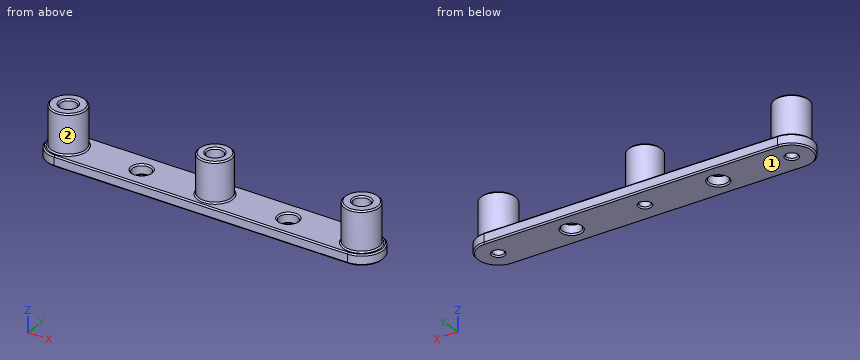
```python
from build123d import *

# Parameters (mm, degrees)
F0_R     = 3.5
F1_DEPTH = 4
F2_R     = 6.5
F2_R_2   = 6.15
F3_DEPTH = 15
F4_R     = 2
F5_DEPTH = 25
F6_R     = 3.05
F7_DEPTH = 6
F8_SIZE  = 0.5


with BuildPart() as f1:
    # F0 (on Top) → F1 (new body)
    with BuildSketch(Plane.XY):
        with BuildLine():
            Line((-56, -8), (56, -8))
            ThreePointArc((56, -8), (64, 0), (56, 8))
            Line((56, 8), (-56, 8))
            ThreePointArc((-56, 8), (-64, 0), (-56, -8))
        make_face()
        with Locations((-28, 0)):
            Circle(F0_R, mode=Mode.SUBTRACT)
        with Locations((28, 0)):
            Circle(F0_R, mode=Mode.SUBTRACT)
    extrude(amount=F1_DEPTH)

    # F2 (on face) → F3 (join)
    with BuildSketch(Plane.XY.offset(4)):
        with Locations((-56, 0)):
            Circle(F2_R)
        with Locations((56, 0)):
            Circle(F2_R)
        Circle(F2_R_2)
    extrude(amount=F3_DEPTH)

    # F4 (on face) → F5 (cut)
    with BuildSketch(Plane.XY.offset(19)):
        with Locations((56, 0)):
            Circle(F4_R)
        Circle(F4_R)
        with Locations((-56, 0)):
            Circle(F4_R)
    extrude(amount=-F5_DEPTH, mode=Mode.SUBTRACT)

    # F6 (on face) → F7 (cut)
    with BuildSketch(Plane.XY.offset(19)):
        with Locations((-56, 0)):
            Circle(F6_R)
        Circle(F6_R)
        with Locations((56, 0)):
            Circle(F6_R)
    extrude(amount=-F7_DEPTH, mode=Mode.SUBTRACT)

    # F8
    f8_edges = [f1.edges().sort_by_distance(p)[0] for p in [
        (-62.5, 0, 19),
        (-59.05, 0, 19),
        (-6.15, 0, 19),
        (-3.05, 0, 19),
        (49.5, 0, 19),
        (52.95, 0, 19),
        (-64, 0, 4),
        (0, 8, 4),
        (0, -8, 4),
        (64, 0, 4),
        (-62.5, 0, 4),
        (-31.5, 0, 4),
        (-6.15, 0, 4),
        (24.5, 0, 4),
        (49.5, 0, 4),
        (-64, 0, 0),
        (0, 8, 0),
        (0, -8, 0),
        (64, 0, 0),
        (-58, 0, 0),
        (-31.5, 0, 0),
        (-2, 0, 0),
        (24.5, 0, 0),
        (54, 0, 0),
        (-58, 0, 13),
        (-2, 0, 13),
        (54, 0, 13),
    ]]
    chamfer(f8_edges, length=F8_SIZE)


solid = f1.part
```
Source: CAD feature listing. Evaluate the final solid. Frame: model axes, mm. Face numbers are marked on the shaded views. Coordinates: 2 decimals unless noted, no trailing zeros. Loops run counter-clockwise (first coordinate to the right, second up) from the corner with the lowest first, then second, coordinate; pieces in that order, holes last. Notation, with made-up numbers: (32.25, -8) -> (87.25, -8) arc R15 cw to (87.25, 2) -> close; hole circle Ø11 at (62, 9). An arc over 180 degrees is marked (long way). One line per item, written item: value. Start each with the question number.
Q1. Section query C-C, the plane y = 0. Give the number of separate pieces and of enclosed holes in the cut face, and give its area (3 significant figures).
Q2. Line query: line 1 along Y through (x, z) = (-28, 2.25); line 2 along Y through (x, z) = (-56, 15); line 3 along X through (y, z) = (4, 14.5). Output: solid intervals per line, ascending.
Q3. Section query A-A, the plane x = 28. Return the cut outline in (y, z).
Q4. Section query B-B, the plane z = 7. Return the cut outline in (x, y), and give its area (3 significant figures).
Q5. Contact query for flat-ended pins moving along their axis: P1, Ø5.5, axis at x = -56, y = 0, coming from the +Z side; P2, Ø1.5, axis at y = -4, z = 11, coming from the -X side; P3, Ø5, axis at y = 1.5, z = 7, coming from the -X side; P4, Ø7, axis at x = 0, y = 0, coming from the -Z side. Output: stop coordinate, or through.
Q6. Mould query, pull axis X, two halves, no side actions, for the marked faces 1 and 2. Classes: pulls with the +X half, pulls with the -X half, needs draft (parallel to the pull), parting line crosses it, or undercut.
Results:
1. separate pieces: 6
1. enclosed holes: 0
1. area: 761 mm^2
2. line 1: -8 to -3.5, 3.5 to 8
2. line 2: -6.5 to -3.05, 3.05 to 6.5
2. line 3: -61.12 to -50.88, -4.67 to 4.67, 50.88 to 61.12
3. outline: (-8, 0.5) -> (-7.5, 0) -> (-4, 0) -> (-3.5, 0.5) -> (-3.5, 3.5) -> (-4, 4) -> (-7.5, 4) -> (-8, 3.5) -> close; (3.5, 0.5) -> (4, 0) -> (7.5, 0) -> (8, 0.5) -> (8, 3.5) -> (7.5, 4) -> (4, 4) -> (3.5, 3.5) -> close
4. outline: circle Ø13 at (-56, 0); circle Ø12.3 at (0, 0); circle Ø13 at (56, 0); hole circle Ø4 at (-56, 0); hole circle Ø4 at (0, 0); hole circle Ø4 at (56, 0)
4. area: 347 mm^2
5. P1: z = 13
5. P2: x = -61.63
5. P3: x = -62.5
5. P4: z = 0
6. face 1: needs draft
6. face 2: undercut
